```python
from build123d import *

# Parameters (mm, degrees)
REVOLVE_1_ANGLE              = 180
SKETCH_6_W                   = 6.5
SKETCH_6_H                   = 146.9
HOLE_WIZARD_M8_1_D           = 6.8
HOLE_WIZARD_M8_1_DEPTH       = 19.75
HOLE_WIZARD_M8_1_CSINK_D     = 8.05
HOLE_WIZARD_M8_1_CSINK_ANGLE = 90
HOLE_WIZARD_M8_1_TIP         = 2.042926105


with BuildPart() as part:
    # 草图1 → 旋转1 (revolve)
    with BuildSketch(Plane(origin=(0, 0, 0), x_dir=(1, 0, 0), z_dir=(0, 1, 0))):
        with BuildLine():
            Line((0, 7.75), (0, -7.75))
            ThreePointArc((0, -7.75), (7.75, 0), (0, 7.75))
        make_face()
    revolve(axis=Axis((0, 0, -7.75), (0, 0, 1)), revolution_arc=REVOLVE_1_ANGLE)

    # 草图6 → 旋转2 (revolve)
    with BuildSketch(Plane(origin=(0, 0, 0), x_dir=(0, 0, -1), z_dir=(1, 0, 0)), mode=Mode.PRIVATE) as revolve_2_sk:
        with Locations((3.25, -73.45)):
            Rectangle(SKETCH_6_W, SKETCH_6_H)
    revolve(revolve_2_sk.sketch.rotate(Axis((0, 0, 0), (0, -1, 0)), 180), axis=Axis((0, 0, 0), (0, -1, 0)))

    # M8 螺纹孔1
    with Locations(Plane(origin=(0, -146.9, 0), x_dir=(0, 0, -1), z_dir=(0, -1, 0))):
        with Locations((0, 0)):
            CounterSinkHole(HOLE_WIZARD_M8_1_D / 2, HOLE_WIZARD_M8_1_CSINK_D / 2, depth=HOLE_WIZARD_M8_1_DEPTH, counter_sink_angle=HOLE_WIZARD_M8_1_CSINK_ANGLE)
            with Locations((0, 0, -(HOLE_WIZARD_M8_1_DEPTH + HOLE_WIZARD_M8_1_TIP / 2))):  # 118° drill point
                Cone(0, HOLE_WIZARD_M8_1_D / 2, HOLE_WIZARD_M8_1_TIP, mode=Mode.SUBTRACT)


solid = part.part
```
Can you work these out from the model? Positions are in its coordinate system, mm. Round coordinates to 2 decimals unless told otherwise and drop trailing zeros. Loops run counter-clockwise (first coordinate to the right, second up) from the corner with the lowest first, then second, coordinate; pieces in that order, holes last.
Item 1: If we mould it in two halves opening along Z, with no side actions, what happens to faces 1 (the flat face through (-3, -146.9, -3)), 2 (the conical face through (-0.576, -125.462, 0.128)), 3 (the cylindrical face through (3.955, -72.422, -5.158))? For each: +Z half, -Z half, draft (parallel to the pull), parting line (faces both ways), or undercut.
Item 2: Will these pins go through, and if not, where does the flat tip stop? pin 1 Ø2 at (y, z) = (-31.5, 5.5) entering from -X; pin 2 Ø2 at (y, z) = (-49, -4.5) entering from +X; pin 3 Ø3 at (y, z) = (-33, 0) entering from +X.
Item 3: Please list where these lines run through material, in increasing order: L1, parallel to X at y = -137, z = 0; L2, parallel to Z at x = -0.5, y = -71.
Item 4: Suppose I cut it at A-A, the plane y = -94.5. Write out the boundary of the cut face in (x, z), then the cut area to 3 significant figures.
Reported:
1. face 1: draft
1. face 2: undercut
1. face 3: parting line
2. pin 1: stops at x = -4.69
2. pin 2: stops at x = 5.48
2. pin 3: stops at x = 6.5
3. L1: x = -6.5 to -3.4, 3.4 to 6.5
3. L2: z = -6.48 to 6.48
4. outline: circle Ø13 at (0, 0)
4. area: 133 mm2
